The listing builds one solid part. Answer for the finished solid, in the listing's coordinates (mm). Coordinates: 2 decimals unless noted, no trailing zeros. Order: outer loops, then holes, each group sorted by start corner. A loop starts at its lowest first (then second) coordinate and runs counter-clockwise, first axis right, second up. Notation, with made-up numbers: (-21, 25) -> (-13, 25) arc R14 ccw to (-13, 43) -> close; hole circle Ø6 at (-27, 13.25). An arc over 180 degrees is marked (long way). Answer in a Markdown table with one row per item.
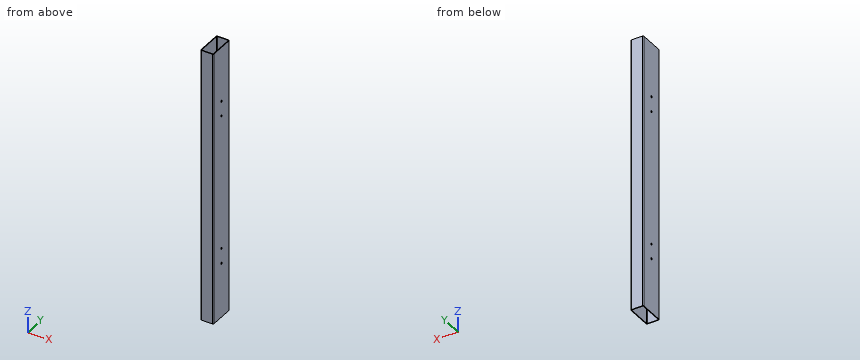
```python
from build123d import *

# Parameters (mm, degrees)
EXTRUDE_THIN1_DEPTH      = 640
EXTRUDE_THIN1_DEPTH_BACK = 640
CUT_EXTRUDE1_DEPTH       = 644.506021728
CUT_EXTRUDE1_DEPTH_BACK  = 644.506021728
SKETCH2_R                = 5


with BuildPart() as part:
    # Sketch1 → Extrude-Thin1 (new, two sides: drawn at the far end of the back side and taken through both)
    with BuildSketch(Plane.XY.offset(-EXTRUDE_THIN1_DEPTH_BACK)):
        with BuildLine():
            Line((-30, 55), (-30, -55))
            ThreePointArc((-30, -55), (-28.535533906, -58.535533906), (-25, -60))
            Line((-25, -60), (25, -60))
            ThreePointArc((25, -60), (28.535533906, -58.535533906), (30, -55))
            Line((30, -55), (30, 55))
            ThreePointArc((30, 55), (28.535533906, 58.535533906), (25, 60))
            Line((25, 60), (-25, 60))
            ThreePointArc((-25, 60), (-28.535533906, 58.535533906), (-30, 55))
        make_face()
        with BuildLine():
            Line((-27, 55), (-27, -55))
            ThreePointArc((-27, -55), (-26.414213562, -56.414213562), (-25, -57))
            Line((-25, -57), (25, -57))
            ThreePointArc((25, -57), (26.414213562, -56.414213562), (27, -55))
            Line((27, -55), (27, 55))
            ThreePointArc((27, 55), (26.414213562, 56.414213562), (25, 57))
            Line((25, 57), (-25, 57))
            ThreePointArc((-25, 57), (-26.414213562, 56.414213562), (-27, 55))
        make_face(mode=Mode.SUBTRACT)
    extrude(amount=EXTRUDE_THIN1_DEPTH + EXTRUDE_THIN1_DEPTH_BACK)

    # Sketch2 → Cut-Extrude1 (cut, two sides: drawn at the far end of the back side and taken through both)
    with BuildSketch(Plane(origin=(0, 0, 0), x_dir=(0, 0, -1), z_dir=(1, 0, 0)).offset(-CUT_EXTRUDE1_DEPTH_BACK)):
        with Locations((-314.25, 0)):
            Circle(SKETCH2_R)
        with Locations((-385.25, 0)):
            Circle(SKETCH2_R)
        with Locations((314.25, 0)):
            Circle(SKETCH2_R)
        with Locations((385.25, 0)):
            Circle(SKETCH2_R)
    extrude(amount=CUT_EXTRUDE1_DEPTH + CUT_EXTRUDE1_DEPTH_BACK, mode=Mode.SUBTRACT)


solid = part.part
```
(1) Find the intervals of material crossed by line 1 along Z through (x, y) = (-28, 0); line 2 along Y through (x, z) = (-1.5, -232.5); line 3 along X through (y, z) = (41.5, 446), in increasing order. Write a range as from..to.
Check values:
| item | result |
|---|---|
| line 1 | -640..-390.25, -380.25..-319.25, -309.25..309.25, 319.25..380.25, 390.25..640 |
| line 2 | -60..-57, 57..60 |
| line 3 | -30..-27, 27..30 |
(2) A cutting plane is placed at C-C, the plane z = 29.5. Determine the outline of the cut face in (x, y), then the cut area to 3 significant figures.
Check values:
| item | result |
|---|---|
| outline | (-30, -55) arc R5 ccw to (-25, -60) -> (25, -60) arc R5 ccw to (30, -55) -> (30, 55) arc R5 ccw to (25, 60) -> (-25, 60) arc R5 ccw to (-30, 55) -> close; hole (-27, -55) arc R2 ccw to (-25, -57) -> (25, -57) arc R2 ccw to (27, -55) -> (27, 55) arc R2 ccw to (25, 57) -> (-25, 57) arc R2 ccw to (-27, 55) -> close |
| area | 1,030 mm² |
(3) A cutting plane is placed at A-A, the plane y = -33. Determine the outline of the cut face in (x, z).
Check values:
| item | result |
|---|---|
| outline | (-30, -640) -> (-27, -640) -> (-27, 640) -> (-30, 640) -> close; (27, -640) -> (30, -640) -> (30, 640) -> (27, 640) -> close |
(4) A cutting plane is placed at B-B, the plane x = 16. Determine the outline of the cut face in (y, z), then the cut area to 3 significant figures.
Check values:
| item | result |
|---|---|
| outline | (-60, -640) -> (-57, -640) -> (-57, 640) -> (-60, 640) -> close; (57, -640) -> (60, -640) -> (60, 640) -> (57, 640) -> close |
| area | 7,680 mm² |
